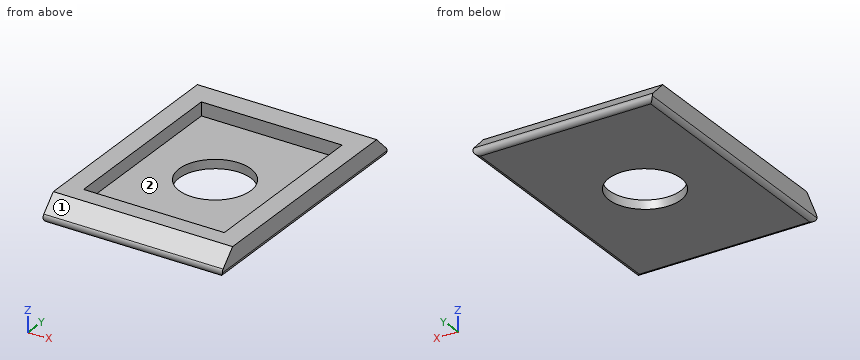
```python
from build123d import *

# Parameters (mm, degrees)
PAD031_DEPTH    = 10
SKETCH069_W     = 15.7
SKETCH069_H     = 20.45
POCKET022_DEPTH = 1.5
FILLET010_R     = 0.5
SKETCH083_R     = 4
POCKET024_DEPTH = 4.001


with BuildPart() as part:
    # Sketch068 → Pad031 (new body, symmetric)
    with BuildSketch(Plane.YZ):
        Polygon((-15, -4), (15, -4), (12.5, -1.5), (-12.5, -1.5), align=None)
    extrude(amount=PAD031_DEPTH, both=True)

    # Sketch069 → Pocket022 (cut)
    with BuildSketch(Plane(origin=(0, 2, -1.5), x_dir=(1, 0, 0), z_dir=(0, 0, 1))):
        with Locations((0, -2.375)):
            Rectangle(SKETCH069_W, SKETCH069_H)
    extrude(amount=-POCKET022_DEPTH, mode=Mode.SUBTRACT)

    # Fillet010
    fillet010_edges = [part.edges().sort_by_distance(p)[0] for p in [
        (0, -15, -4),
        (0, 15, -4),
        (-10, 0, -4),
        (10, 0, -4),
    ]]
    fillet(fillet010_edges, radius=FILLET010_R)

    # Sketch083 → Pocket024 (cut, through all)
    with BuildSketch(Plane.XY):
        Circle(SKETCH083_R)
    extrude(amount=-POCKET024_DEPTH, mode=Mode.SUBTRACT)


with BuildPart() as part_1:
    # Body022 placement: moved
    add(part.part.moved(Location((0, -2, 2.5))))


solid = part_1.part
```
Input: part model. Units: mm. Frame: model coordinates. Face numbers are marked on the shaded views. Give positions to 0.01 mm unless a question says otherwise; leave off trailing zeros. Order: outer loops, then holes, each group sorted by start corner. A loop starts at its lowest first (then second) coordinate and runs counter-clockwise, first axis right, second up.
1. Cut plane D-D (y = 3.5). Return loops of the section in (x, z).
Computed:
outline: (-10, -1) arc R0.5 ccw to (-9.5, -1.5) - (9.5, -1.5) arc R0.5 ccw to (10, -1) - (10, 1) - (7.85, 1) - (7.85, -0.5) - (-7.85, -0.5) - (-7.85, 1) - (-10, 1) - close
2. Cut plane C-C (z = 0.25). Return loops of the section in (x, y).
Computed:
outline: (-10, -15.25) - (10, -15.25) - (10, 11.25) - (-10, 11.25) - close; hole (-7.85, -12.6) - (7.85, -12.6) - (7.85, 7.85) - (-7.85, 7.85) - close
3. Pin query (flat end, axial travel): pin 1 Ø1 at (x, y) = (-3.5, -9) entering from +Z. Return the tip coordinate at first contact, or that it passes through.
Computed:
pin 1: stops at z = -0.5
4. Line query: probe 1 along X at (y, z) = (4.5, 0); probe 2 along Z at (x, y) = (1.25, -8.75); probe 3 along Y at (x, z) = (0, -0.7). Output: solid intervals per line, ascending.
Computed:
probe 1: x = -10 to -7.85, 7.85 to 10
probe 2: z = -1.5 to -0.5
probe 3: y = -16.19 to -6, 2 to 12.19
5. Cut plane A-A (x = 0). Return loops of the section in (y, z).
Computed:
outline: (-16.15, -0.65) arc R0.5 ccw to (-15.79, -1.5) - (-6, -1.5) - (-6, -0.5) - (-12.6, -0.5) - (-12.6, 1) - (-14.5, 1) - close; (2, -1.5) - (11.79, -1.5) arc R0.5 ccw to (12.15, -0.65) - (10.5, 1) - (7.85, 1) - (7.85, -0.5) - (2, -0.5) - close
6. Cut plane B-B (y = -2). Return loops of the section in (x, z).
Computed:
outline: (-10, -1) arc R0.5 ccw to (-9.5, -1.5) - (-4, -1.5) - (-4, -0.5) - (-7.85, -0.5) - (-7.85, 1) - (-10, 1) - close; (4, -1.5) - (9.5, -1.5) arc R0.5 ccw to (10, -1) - (10, 1) - (7.85, 1) - (7.85, -0.5) - (4, -0.5) - close
7. Draft query along X for the marked faces 1 and 2. Return one class per face: released by +X, released by -X, zero draft, split by the parting line, or undercut.
Computed:
face 1: zero draft
face 2: undercut
